Print and shaded views of the part. All mm, measured from the part's lowest x, y and z. A direction names the side the tool comes from. Coordinates: 2 decimals unless noted, no trailing zeros. Write each loop counter-clockwise with the first axis right and the second up, starting at its lowest first coordinate (ties: lowest second). Pieces come first, ordered by that corner, then holes. Notation, with made-up numbers: (59, 39) -> (63, 39) arc R27 cw to (63, 75) -> close; hole circle Ø8 at (-15, -4). An arc over 180 degrees is marked (long way). Write item = value, one per line.
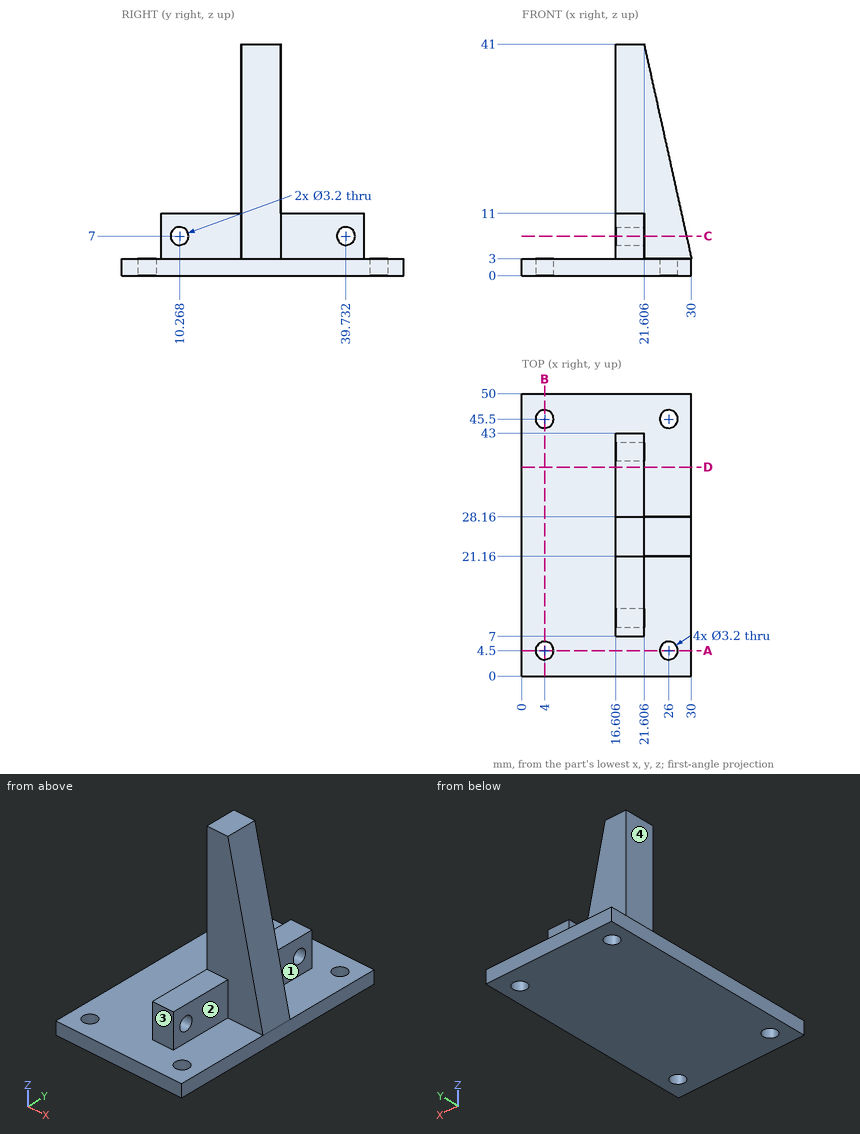
Q1. Pin check, flat tips, straight feed: pin 1 (1 mm diameter, centred on x = 19, y = 9, fed in from +Z); pin 2 (10 mm diameter, centred on x = 12.5, z = 21, fed in from -Y); pin 3 (15 mm diameter, centred on x = 21.5, y = 31.5, fed in from +Z); pin 4 (1.9 mm diameter, centred on x = 4, y = 4.5, fed in from -Z). Stop position of each tip, or through.
Model answer:
pin_1 = 11
pin_2 = 21.16
pin_3 = 41
pin_4 = through
Q2. Saw through at B-B on x = 4. Give the cut face in (y, z), and give its area (3 significant figures).
Model answer:
outline = (0, 0) -> (2.9, 0) -> (2.9, 3) -> (0, 3) -> close; (6.1, 0) -> (43.9, 0) -> (43.9, 3) -> (6.1, 3) -> close; (47.1, 0) -> (50, 0) -> (50, 3) -> (47.1, 3) -> close
area = 131 mm²
Q3. Saw through at C-C on z = 7. Give the cut face in (x, y).
Model answer:
outline = (16.61, 7) -> (21.61, 7) -> (21.61, 8.67) -> (16.61, 8.67) -> close; (16.61, 11.87) -> (21.61, 11.87) -> (21.61, 21.16) -> (29.12, 21.16) -> (29.12, 28.16) -> (21.61, 28.16) -> (21.61, 38.13) -> (16.61, 38.13) -> close; (16.61, 41.33) -> (21.61, 41.33) -> (21.61, 43) -> (16.61, 43) -> close
Q4. Which spindle directions (+Z, -Z, +X, -X, +Y, -Y) get a long thin tool onto all of the face, cutting with end or side? Do the marked faces 1, 2, 3 and 4. Say none if no direction does.
Model answer:
face_1 = +Z, +X, +Y
face_2 = +Z, +X, -Y
face_3 = +Z, +X, -X, -Y
face_4 = +Z, -X, +Y, -Y
Q5. Saw through at D-D on y = 37. Give the cut face in (x, z), and give its area (3 significant figures).
Model answer:
outline = (0, 0) -> (30, 0) -> (30, 3) -> (21.61, 3) -> (21.61, 11) -> (16.61, 11) -> (16.61, 3) -> (0, 3) -> close
area = 130 mm²
Q6. Probe line 1 (Y direction, x = 4, z = 1.1); line 2 (X direction, y = 45, z = 1); line 3 (Y direction, x = 26.5, z = 13). List the from-to ranges inside material, lowest first. Write a range as from..to.
Model answer:
line_1 = 0..2.9, 6.1..43.9, 47.1..50
line_2 = 0..2.48, 5.52..24.48, 27.52..30
line_3 = 21.16..28.16
Q7. Saw through at A-A on y = 4.5. Give the cut face in (x, z), and give its area (3 significant figures).
Model answer:
outline = (0, 0) -> (2.4, 0) -> (2.4, 3) -> (0, 3) -> close; (5.6, 0) -> (24.4, 0) -> (24.4, 3) -> (5.6, 3) -> close; (27.6, 0) -> (30, 0) -> (30, 3) -> (27.6, 3) -> close
area = 70.8 mm²
